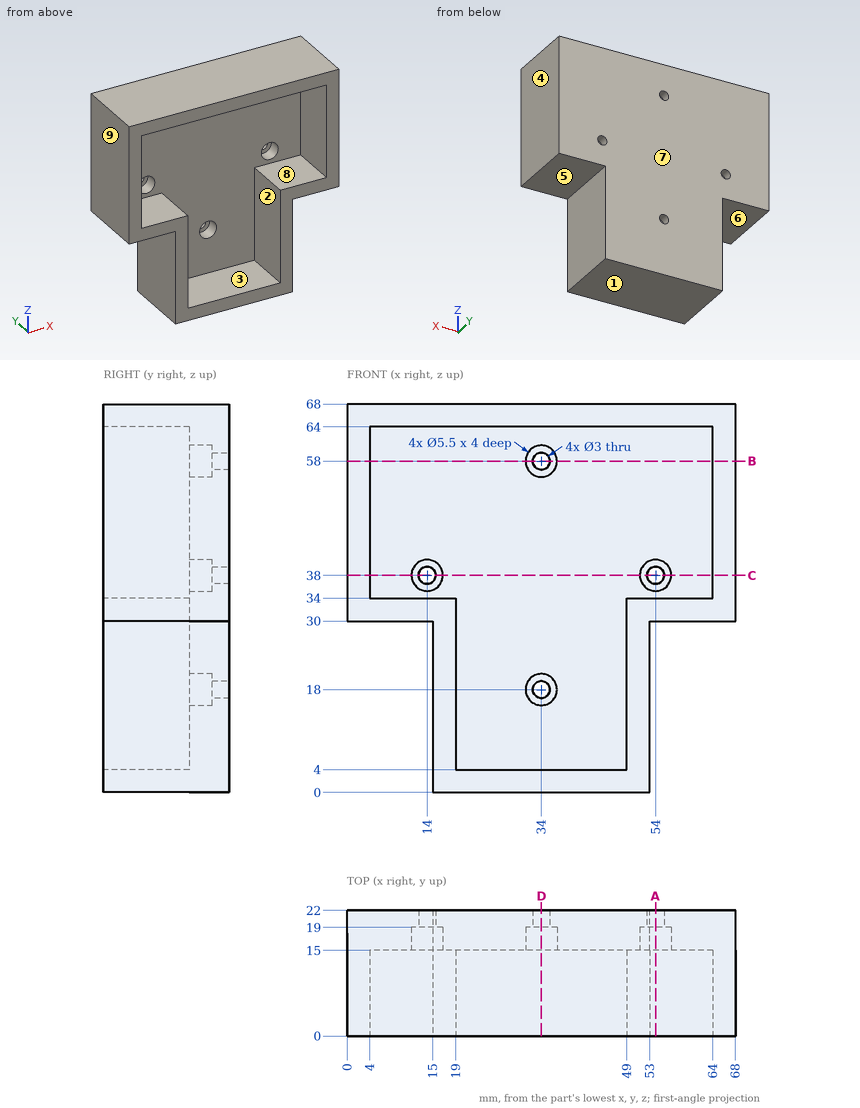
Print and shaded views of the part. All mm, measured from the part's lowest x, y and z. A direction names the side the tool comes from. Round coordinates to 2 decimals unless told otherwise and drop trailing zeros. Loops run counter-clockwise (first coordinate to the right, second up) from the corner with the lowest first, then second, coordinate; pieces in that order, holes last. Notation, with made-up numbers: (15, 42) -> (68, 42) arc R17 ccw to (68, 47) -> close; hole circle Ø9 at (-37.5, 4). An arc over 180 degrees is marked (long way). Use CSV: the item, a comma, the result in double quotes. Start each with the question number.
1) Cut at D-D, the plane x = 34. Write the cut outline in (y, z), plus the area to 3 significant figures.
2) Cut at C-C, the plane z = 38. Write the cut outline in (x, y), plus the area to 3 significant figures.
3) Wall check: L1, parallel to X at y = 17, z = 18; L2, parallel to X at y = 6.5, z = 39; L3, parallel to X at y = 17.7, z = 38. Give the ranges that are in metal, low to high. Write a range as [from, to].
4) Pull direction X, two halves, no side cores. Call the marked faces 1, 2, 3 and 4: +X half, -X half, draft (parallel to the pull), parting line (faces both ways), or undercut.
5) Cut at A-A, the plane x = 54. Write the cut outline in (y, z).
6) Drop flat-ended pins along their axis: P1, Ø1.5, axis at x = 46, y = 5.5, coming from the -Z side; P2, Ø4.5, axis at y = 5.5, z = 26.5, coming from the -X side; P3, Ø12, axis at y = 2.5, z = 15, coming from the +X side; P4, Ø4.5, axis at x = 62, y = 7, coming from the -Z side. Give the stop position or say it passes through.
7) Which spindle directions (+Z, -Z, +X, -X, +Y, -Y) get a long thin tool onto all of the face, cutting with end or side? Do the marked faces 5, 6, 7, 8 and 9. Say none if no direction does.
8) Cut at B-B, the plane z = 58. Write the cut outline in (x, y).
Determined:
1,outline,"(0, 0) -> (22, 0) -> (22, 16.5) -> (19, 16.5) -> (19, 15.25) -> (15, 15.25) -> (15, 4) -> (0, 4) -> close; (0, 64) -> (15, 64) -> (15, 60.75) -> (19, 60.75) -> (19, 59.5) -> (22, 59.5) -> (22, 68) -> (0, 68) -> close; (15, 20.75) -> (19, 20.75) -> (19, 19.5) -> (22, 19.5) -> (22, 56.5) -> (19, 56.5) -> (19, 55.25) -> (15, 55.25) -> close"
1,area,"534 mm2"
2,outline,"(0, 0) -> (4, 0) -> (4, 15) -> (11.25, 15) -> (11.25, 19) -> (12.5, 19) -> (12.5, 22) -> (0, 22) -> close; (15.5, 19) -> (16.75, 19) -> (16.75, 15) -> (51.25, 15) -> (51.25, 19) -> (52.5, 19) -> (52.5, 22) -> (15.5, 22) -> close; (55.5, 19) -> (56.75, 19) -> (56.75, 15) -> (64, 15) -> (64, 0) -> (68, 0) -> (68, 22) -> (55.5, 22) -> close"
2,area,"534 mm2"
3,L1,"x = [15, 31.25], [36.75, 53]"
3,L2,"x = [0, 4], [64, 68]"
3,L3,"x = [0, 11.25], [16.75, 51.25], [56.75, 68]"
4,face 1,"draft"
4,face 2,"undercut"
4,face 3,"undercut"
4,face 4,"+X half"
5,outline,"(0, 30) -> (22, 30) -> (22, 36.5) -> (19, 36.5) -> (19, 35.25) -> (15, 35.25) -> (15, 34) -> (0, 34) -> close; (0, 64) -> (15, 64) -> (15, 40.75) -> (19, 40.75) -> (19, 39.5) -> (22, 39.5) -> (22, 68) -> (0, 68) -> close"
6,P1,"stops at z = 0"
6,P2,"stops at x = 15"
6,P3,"stops at x = 53"
6,P4,"stops at z = 30"
7,face 5,"-Z, +X, +Y, -Y"
7,face 6,"-Z, -X, +Y, -Y"
7,face 7,"+Z, -Z, +X, -X, +Y"
7,face 8,"-Y"
7,face 9,"+Z, -Z, -X, +Y, -Y"
8,outline,"(0, 0) -> (4, 0) -> (4, 15) -> (31.25, 15) -> (31.25, 19) -> (32.5, 19) -> (32.5, 22) -> (0, 22) -> close; (35.5, 19) -> (36.75, 19) -> (36.75, 15) -> (64, 15) -> (64, 0) -> (68, 0) -> (68, 22) -> (35.5, 22) -> close"
